```python
from build123d import *

# Parameters (mm, degrees)
EXTRUDE1_DEPTH            = 5.3
EXTRUDE1_DEPTH_BACK       = 10
SKETCH1_W                 = 34
SKETCH1_H                 = 38.5
SKETCH5_W                 = 32
SKETCH5_H                 = 36.5
CUT_EXTRUDE2_DEPTH        = 2
CUT_EXTRUDE3_DEPTH        = 0.2
CUT_EXTRUDE3_DEPTH_BACK   = 11.3
SKETCH6_W                 = 30.4
SKETCH6_H                 = 34.9
FILLET1_R                 = 2
SKETCH11_W                = 30.4
SKETCH11_H                = 4
EXTRUDE4_DEPTH            = 11
F_1_CLEARANCE_HOLE1_D     = 2.0574
F_1_CLEARANCE_HOLE1_DEPTH = 8
F_1_CLEARANCE_HOLE1_TIP   = 0.618105319
SKETCH17_R                = 3
CUT_EXTRUDE6_DEPTH        = 10
SKETCH18_W                = 3
SKETCH18_H                = 3
EXTRUDE5_DEPTH            = 2.3
SKETCH19_W                = 8.3
SKETCH19_H                = 3.2
CUT_EXTRUDE7_DEPTH        = 3
SKETCH20_R                = 8.5
EXTRUDE6_DEPTH            = 6
SKETCH21_R                = 6.6
CUT_EXTRUDE8_DEPTH        = 6
SKETCH22_R                = 4.45
EXTRUDE7_DEPTH            = 6
SKETCH23_R                = 3
CUT_EXTRUDE9_DEPTH        = 6
FILLET2_R                 = 1
FILLET3_R                 = 1
FILLET4_R                 = 1
FILLET5_R                 = 1
FILLET6_R                 = 2
FILLET7_R                 = 1


with BuildPart() as part:
    # Sketch1 → Extrude1 (new, two sides: drawn at the far end of the back side and taken through both)
    with BuildSketch(Plane.XY.offset(-EXTRUDE1_DEPTH_BACK)):
        with Locations((8.75, 17)):
            Rectangle(SKETCH1_W, SKETCH1_H)
    extrude(amount=EXTRUDE1_DEPTH + EXTRUDE1_DEPTH_BACK)

    # Sketch5 → Cut-Extrude2 (cut)
    with BuildSketch(Plane.XY.offset(5.3)):
        with Locations((8.75, 17)):
            Rectangle(SKETCH5_W, SKETCH5_H)
    extrude(amount=-CUT_EXTRUDE2_DEPTH, mode=Mode.SUBTRACT)

    # Sketch6 → Cut-Extrude3 (cut, two sides: drawn at the far end of the back side and taken through both)
    with BuildSketch(Plane.XY.offset(3.3).offset(-CUT_EXTRUDE3_DEPTH_BACK)):
        with Locations((8.75, 17)):
            Rectangle(SKETCH6_W, SKETCH6_H)
    extrude(amount=CUT_EXTRUDE3_DEPTH + CUT_EXTRUDE3_DEPTH_BACK, mode=Mode.SUBTRACT)

    # Fillet1
    fillet1_edges = [part.edges().sort_by_distance(p)[0] for p in [
        (-8.25, 17, -10),
        (8.75, 36.25, -10),
        (25.75, 17, -10),
        (8.75, -2.25, -10),
        (-8.25, 36.25, -2.35),
        (25.75, 36.25, -2.35),
        (25.75, -2.25, -2.35),
        (-8.25, -2.25, -2.35),
    ]]
    fillet(fillet1_edges, radius=FILLET1_R)

    # Sketch11 → Extrude4 (add)
    with BuildSketch(Plane.XY.offset(-8)):
        with Locations((8.75, 32.45)):
            Rectangle(SKETCH11_W, SKETCH11_H)
    extrude(amount=EXTRUDE4_DEPTH)

    # #1 Clearance Hole1
    with Locations(Plane.XY.offset(3.3)):
        with Locations((-4.45, 32.45)):
            Hole(F_1_CLEARANCE_HOLE1_D / 2, depth=F_1_CLEARANCE_HOLE1_DEPTH)
            with Locations((0, 0, -(F_1_CLEARANCE_HOLE1_DEPTH + F_1_CLEARANCE_HOLE1_TIP / 2))):  # 118° drill point
                Cone(0, F_1_CLEARANCE_HOLE1_D / 2, F_1_CLEARANCE_HOLE1_TIP, mode=Mode.SUBTRACT)

    # Sketch17 → Cut-Extrude6 (cut)
    with BuildSketch(Plane(origin=(0, 0, -10), x_dir=(-1, 0, 0), z_dir=(0, 0, -1))):
        with Locations((-8.75, 15)):
            Circle(SKETCH17_R)
    extrude(amount=-CUT_EXTRUDE6_DEPTH, mode=Mode.SUBTRACT)

    # Sketch18 → Extrude5 (add)
    with BuildSketch(Plane.XY.offset(-8)):
        with Locations((-4.95, 28.95)):
            Rectangle(SKETCH18_W, SKETCH18_H)
    extrude(amount=EXTRUDE5_DEPTH)

    # Sketch19 → Cut-Extrude7 (cut)
    with BuildSketch(Plane.XZ.offset(2.25)):
        with Locations((17.9, -6.4)):
            Rectangle(SKETCH19_W, SKETCH19_H)
    extrude(amount=-CUT_EXTRUDE7_DEPTH, mode=Mode.SUBTRACT)

    # Sketch20 → Extrude6 (add)
    with BuildSketch(Plane(origin=(0, 0, -10), x_dir=(-1, 0, 0), z_dir=(0, 0, -1))):
        with Locations(Location((-8.75, 15, 0), (0, 0, 180))):
            Circle(SKETCH20_R)
    extrude(amount=EXTRUDE6_DEPTH)

    # Sketch21 → Cut-Extrude8 (cut)
    with BuildSketch(Plane(origin=(0, 0, -16), x_dir=(-1, 0, 0), z_dir=(0, 0, -1))):
        with Locations((-8.75, 15)):
            Circle(SKETCH21_R)
    extrude(amount=-CUT_EXTRUDE8_DEPTH, mode=Mode.SUBTRACT)

    # Sketch22 → Extrude7 (add)
    with BuildSketch(Plane(origin=(0, 0, -10), x_dir=(-1, 0, 0), z_dir=(0, 0, -1))):
        with Locations((-8.75, 15)):
            Circle(SKETCH22_R)
    extrude(amount=EXTRUDE7_DEPTH)

    # Sketch23 → Cut-Extrude9 (cut)
    with BuildSketch(Plane(origin=(0, 0, -16), x_dir=(-1, 0, 0), z_dir=(0, 0, -1))):
        with Locations((-8.75, 15)):
            Circle(SKETCH23_R)
    extrude(amount=-CUT_EXTRUDE9_DEPTH, mode=Mode.SUBTRACT)

    # Fillet2
    fillet2_edges = [part.edges().sort_by_distance(p)[0] for p in [
        (15.35, 15, -16),
    ]]
    fillet(fillet2_edges, radius=FILLET2_R)

    # Fillet3
    # the kernel refuses this fillet: 1 mm, written as the material it takes off along each edge
    with BuildSketch(Plane(origin=(8.75, 15, -16), x_dir=(1, 0, 0), z_dir=(0, 1, 0))) as fillet3_piece_1:
        with BuildLine():
            CenterArc((7.5, -0.994987437), FILLET3_R, 0, 84.260829523)
            Line((8.5, -0.994987437), (8.52, -0.994987437))
            Line((8.52, -0.994987437), (8.52, 0))
            Line((8.52, 0), (8.5, 0.02))
            ThreePointArc((8.5, 0.02), (8.05, 0.02), (7.602, 0.019899749))
            Line((7.602, 0.019899749), (7.6, 0))
        make_face()
    revolve(axis=Axis((8.75, 15, -16), (0, 0, -1)), mode=Mode.SUBTRACT)

    # Fillet4
    fillet4_edges = [part.edges().sort_by_distance(p)[0] for p in [
        (11.75, 15, -16),
    ]]
    fillet(fillet4_edges, radius=FILLET4_R)

    # Fillet5
    # the kernel refuses this fillet: 1 mm, written as the material it takes off along each edge
    with BuildSketch(Plane(origin=(8.75, 15, -16), x_dir=(-1, 0, 0), z_dir=(0, -1, 0))) as fillet5_piece_1:
        with BuildLine():
            CenterArc((3.45, -0.835164654), FILLET5_R, 0, 56.632987031)
            Line((4.45, -0.835164654), (4.47, -0.835164654))
            Line((4.47, -0.835164654), (4.47, 0))
            Line((4.47, 0), (4.45, 0.02))
            ThreePointArc((4.45, 0.02), (4.225, 0.02), (4.011, 0.016703293))
            Line((4.011, 0.016703293), (4, 0))
        make_face()
    revolve(axis=Axis((8.75, 15, -16), (0, 0, -1)), mode=Mode.SUBTRACT)

    # Fillet6
    fillet6_edges = [part.edges().sort_by_distance(p)[0] for p in [
        (0.25, 15, -10),
    ]]
    fillet(fillet6_edges, radius=FILLET6_R)

    # Fillet7
    fillet7_edges = [part.edges().sort_by_distance(p)[0] for p in [
        (13.75, -2.25, -6.4),
        (22.05, -2.25, -6.4),
        (17.9, -2.25, -4.8),
    ]]
    fillet(fillet7_edges, radius=FILLET7_R)


solid = part.part
```
The model under review builds one solid part; all positions refer to its coordinate system, in mm. A direction names the side the tool comes from. Round coordinates to 2 decimals unless told otherwise and drop trailing zeros. Loops run counter-clockwise (first coordinate to the right, second up) from the corner with the lowest first, then second, coordinate; pieces in that order, holes last. Notation, with made-up numbers: (37.25, -28.75) - (91.25, -28.75) arc R31 cw to (91.25, -0.75) - close; hole circle Ø4 at (69.5, 55). An arc over 180 degrees is marked (long way). Use a Markdown table: item, result. Add a question column.
Q1. Insertion check: pin 1 Ø10 at (x, y) = (12, 20.5) entering from -Z; pin 2 Ø8 at (x, z) = (-2, -13) entering from -Y; pin 3 Ø0.9 at (y, z) = (-1, -6.5) entering from +X; pin 4 Ø15 at (x, y) = (8.75, 15) entering from +Z. Each pin has a flat end and moves straight along its axis. Give the tip position at first contact, or say it passes through.
Q2. Add section A-A (z = 2.5). State the section outline as (x, y) points, plus the area to 3 significant figures.
Q3. For probe 1 along Y at (x, z) = (-4.45, -2); probe 2 along Y at (x, z) = (8.75, -13); probe 3 along Y at (x, z) = (4.5, -3.75), list the stretches that pass through material, from the lowest coordinate up.
Q4. The part is to be moulded in two halves that separate along X. For faces 1 (the face through (9.4, 12.07, -11.55)), 2 (the face through (25.15, -1.68, -1.26)), 3 (the face through (-7.68, 17.24, -9.4)), say which applies: pulls with the +X half, pulls with the -X half, needs draft (parallel to the pull), parting line crosses it, or undercut.
Q5. Machinability: for faces 4 (the face through (13.449, -1.965, -6.337)), 5 (the face through (9, -1.25, 4)), 6 (the face through (6.7, 11.05, -12.55)), 7 (the face through (25.15, 35.68, -1.26)), which of the approach directions +Z, -Z, +X, -X, +Y, -Y give a long, thin tool a straight path to every point of the face, cutting with its end or side? Answer none if there is none.
Q6. Add section B-B (z = -14.25). State the section outline as (x, y) points, plus the area to 3 significant figures.
Q7. Add section C-C (y = 3). State the section outline as (x, z) points, plus the area to 3 significant figures.
Worked answers:
| question | item | result |
|---|---|---|
| 1 | pin 1 | z = -16 |
| 1 | pin 2 | y = -1.98 |
| 1 | pin 3 | x = 25.73 |
| 1 | pin 4 | z = -8 |
| 2 | outline | (-8.25, -0.25) arc R2 ccw to (-6.25, -2.25) - (23.75, -2.25) arc R2 ccw to (25.75, -0.25) - (25.75, 34.25) arc R2 ccw to (23.75, 36.25) - (-6.25, 36.25) arc R2 ccw to (-8.25, 34.25) - close; hole (-6.45, -0.45) - (23.95, -0.45) - (23.95, 30.45) - (-6.45, 30.45) - close; hole circle Ø2.06 at (-4.45, 32.45) |
| 2 | area | 363 mm² |
| 3 | probe 1 | -2.25 to -0.45, 30.45 to 31.42, 33.48 to 36.25 |
| 3 | probe 2 | 6.5 to 8.4, 10.55 to 12, 18 to 19.45, 21.6 to 23.5 |
| 3 | probe 3 | -2.25 to -0.45, 30.45 to 36.25 |
| 4 | face 1 | undercut |
| 4 | face 2 | pulls with the +X half |
| 4 | face 3 | pulls with the -X half |
| 5 | face 4 | -Y |
| 5 | face 5 | +Z |
| 5 | face 6 | -Z |
| 5 | face 7 | +Z, -Z, +X, +Y |
| 6 | outline | circle Ø17 at (8.75, 15); circle Ø8.9 at (8.75, 15); hole circle Ø13.2 at (8.75, 15); hole circle Ø6 at (8.75, 15) |
| 6 | area | 124 mm² |
| 7 | outline | (-8.25, -8) arc R2 ccw to (-6.25, -10) - (23.75, -10) arc R2 ccw to (25.75, -8) - (25.75, 5.3) - (24.75, 5.3) - (24.75, 3.3) - (23.95, 3.3) - (23.95, -8) - (-6.45, -8) - (-6.45, 3.3) - (-7.25, 3.3) - (-7.25, 5.3) - (-8.25, 5.3) - close |
| 7 | area | 111 mm² |
